For this review, take the finished solid that the model builds, in its own axes (mm). A direction names the side the tool comes from. Round coordinates to 2 decimals unless told otherwise and drop trailing zeros. Loops run counter-clockwise (first coordinate to the right, second up) from the corner with the lowest first, then second, coordinate; pieces in that order, holes last. Notation, with made-up numbers: M -17,47 L 11,47 A16 cw 11,66 Z; hole C -17,65 d10. An arc over 180 degrees is marked long. One line per question, with ' | ' between items. Start each with the question number.
1) We need section B-B (y = 0). Give the boundary of the cut face in (x, z).
2) We need section A-A (x = 0). Give the boundary of the cut face in (y, z), and give its area (3 significant figures).
3) We need section C-C (z = 12.75). Give the boundary of the cut face in (x, y).
4) For faces 1 (the face through (12.505, 44.375, 15.14)), 2 (the face through (-41.634, 0.717, 14.912)), 3 (the face through (-3, 47, 3)), list the 3-axis set-ups (+Z, -Z, +X, -X, +Y, -Y) from which the entire face can be reached by the end or side of a thin tool; tool diameter is ignored.
5) For pin 1 Ø5 at (x, y) = (-4.5, 50.5) entering from +Z; pin 2 Ø5 at (x, y) = (-16.5, -44) entering from +Z; pin 3 Ø7.5 at (y, z) = (44.5, 19.5) entering from -X; pin 4 Ø2 at (x, y) = (-38, -5) entering from -Z, all flat-tipped, find the tip position at first contact; note any pin that passes through.
6) For probe 1 along Y at (x, z) = (-17.5, 20.25); probe 2 along X at (y, z) = (-40, 10.75); probe 3 along Y at (x, z) = (18, 20.75), list the stretches that pass through material, from the lowest coordinate up. Write a range as from..to.
7) We need section D-D (x = -15.5). Give the boundary of the cut face in (y, z).
8) Mouldability with a two-part tool opening along Y and no side actions: class faces 4 (the face through (25.379, -48.794, 9.547)), 5 (the face through (17, 44, 5)), 6 (the face through (4, -40, 0)), 7 (the face through (-17, 44, 5)) as pulls with the +Y half, pulls with the -Y half, needs draft (parallel to the pull), parting line crosses it, or undercut.
```python
from build123d import *

# Parameters (mm, degrees)
F0_R             = 55
F1_DEPTH         = 25
F3_DEPTH         = 55.001
F3_DEPTH_BACK    = 55.001
F5_DEPTH         = 55.001
F5_DEPTH_BACK    = 55.001
F6_R             = 5
F8_DEPTH         = 20
F8_COPIES2_COUNT = 2


# Not quite as in the source:
# - a pattern or mirror of a feature is missing from the dataset's text; its kind, count and spacing are read off the source's solid


with BuildPart() as f1:
    # F0 (on Top) → F1 (new body)
    with BuildSketch(Plane.XY):
        Circle(F0_R)
        with BuildLine():
            ThreePointArc((39.9217985567, -2.5), (-40, 0), (39.9217985567, 2.5))
            ThreePointArc((39.9217985567, 2.5), (40, 0), (39.9217985567, -2.5))
        make_face(mode=Mode.SUBTRACT)
    extrude(amount=F1_DEPTH)

    # F2 (on Front) → F3 (cut, two sides)
    with BuildSketch(Plane.XZ) as f3_sk:
        Polygon((62.8901384102, 25), (20, 25), (62.8901384102, 5), align=None)
        Polygon((-62.8901384102, 5), (-20, 25), (-62.8901384102, 25), align=None)
    extrude(amount=-F3_DEPTH, mode=Mode.SUBTRACT)
    extrude(f3_sk.sketch, amount=F3_DEPTH_BACK, mode=Mode.SUBTRACT)

    # F4 (on Front) → F5 (cut, two sides)
    with BuildSketch(Plane.XZ) as f5_sk:
        Polygon((11, 25), (-11, 25), (-11, 3), (5, 3), (11, 8), align=None)
    extrude(amount=F5_DEPTH, mode=Mode.SUBTRACT)
    extrude(f5_sk.sketch, amount=-F5_DEPTH_BACK, mode=Mode.SUBTRACT)

    # F6 (on face) → F8 (cut, through all)
    with BuildSketch(Plane.XY.offset(25)):
        with Locations((17.5, 44.1549887905)):
            Circle(F6_R)
    f8 = extrude(amount=-F8_DEPTH, mode=Mode.SUBTRACT)

    # F8_copies: F8 across plane
    add(f8.mirror(Plane(origin=(0, 0, 0), x_dir=(0, 0, -1), z_dir=(-1, 0, 0))), mode=Mode.SUBTRACT)

    # F8_copies1: F8 across plane
    add(f8.mirror(Plane(origin=(0, 0, 0), x_dir=(0, 0, -1), z_dir=(0, -1, 0))), mode=Mode.SUBTRACT)

    # F8_copies2: F8 ×2 about axis
    f8_copies2_axis = Axis((0, 0, 0), (0, 0, 1))
    for i in range(1, F8_COPIES2_COUNT):
        add(f8.rotate(f8_copies2_axis, i * 360 / F8_COPIES2_COUNT), mode=Mode.SUBTRACT)


solid = f1.part
```
Answers below:
1) outline: M -55,0 L -40,0 L -40,15.67 L -55,8.68 Z; M 40,0 L 55,0 L 55,8.68 L 40,15.67 Z
2) outline: M -55,0 L -40,0 L -40,3 L -55,3 Z; M 40,0 L 55,0 L 55,3 L 40,3 Z | area: 90.0 mm^2
3) outline: M -46.27,-29.73 A55 ccw -11,-53.89 L -11,-38.46 A40 cw -11,38.46 L -11,53.89 A55 ccw -46.27,29.73 Z; M 11,-53.89 A55 ccw 46.27,-29.73 L 46.27,29.73 A55 ccw 11,53.89 L 11,38.46 A40 cw 11,-38.46 Z; hole C -17.5,-44.15 d10; hole C -17.5,44.15 d10; hole C 17.5,-44.15 d10; hole C 17.5,44.15 d10
4) face 1: +Z | face 2: +Z, -X, +Y, -Y | face 3: +Z, +Y, -Y
5) pin 1: z = 3 | pin 2: z = 5 | pin 3: x = -36.24 | pin 4: through
6) probe 1: -52.14..-49.15, -39.15..-35.97, 35.97..39.15, 49.15..52.14 | probe 2: -37.75..-20.28, -14.72..-11, 11..14.72, 20.28..37.75 | probe 3: -51.97..-49.13, -39.18..-35.72, 35.72..39.18, 49.13..51.97
7) outline: M -52.77,0 L -36.87,0 L -36.87,25 L -39.57,25 L -39.57,5 L -48.74,5 L -48.74,25 L -52.77,25 Z; M 36.87,0 L 52.77,0 L 52.77,25 L 48.74,25 L 48.74,5 L 39.57,5 L 39.57,25 L 36.87,25 Z
8) face 4: parting line crosses it | face 5: undercut | face 6: needs draft | face 7: undercut
